Input: part model. Units: mm. Frame: model coordinates. A direction names the side the tool comes from. Coordinates: 2 decimals unless noted, no trailing zeros. Write each loop counter-clockwise with the first axis right and the second up, starting at its lowest first coordinate (ties: lowest second). Pieces come first, ordered by that corner, then holes.
1) Pin query (flat end, axial travel): pin 1 Ø6.5 at (x, y) = (59, 17.5) entering from +Z; pin 2 Ø2 at (y, z) = (20, -56.5) entering from -X; pin 3 Ø7 at (x, z) = (-5, -25.5) entering from +Y. Return the tip coordinate at first contact, or that it passes through.
2) Line query: L1, parallel to Z at x = 19, y = 0.5; L2, parallel to Z at x = -30.5, y = 1; L3, parallel to X at y = 36, z = -3. Output: solid intervals per line, ascending.
3) Section query B-B (z = -55). Output: boundary loops of the cut face in (x, y), then the cut area to 3 significant figures.
4) Section query A-A (z = -25.5). Output: boundary loops of the cut face in (x, y).
5) Set-up query: faces 1 (the flat face through (-47, 18, 10)), 2 (the flat face through (30.036, 7.329, -43.679)), 3 (the flat face through (28.017, 4.827, -46.679)). Return all of +Z, -Z, +X, -X, +Y, -Y with unobstructed straight access to the full face (end or side cutting, diameter ignored); none if empty.
6) Section query C-C (x = 6). Output: boundary loops of the cut face in (y, z).
7) Section query D-D (z = 63.5). Output: boundary loops of the cut face in (x, y), then the cut area to 3 significant figures.
8) Draft query along X for faces 4 (the flat face through (39.46, 11.01, 38.78)), 5 (the flat face through (-40, 12, -80.5)), 6 (the cylindrical face through (55.83, 11.62, -46.69)). Return one class per face: pulls with the +X half, pulls with the -X half, needs draft (parallel to the pull), parting line crosses it, or undercut.
from build123d import *

# Parameters (mm, degrees)
BOSS_EXTRUDE1_DEPTH            = 23
BODY_MOVE_COPY1_ANGLE          = 30
BOSS_EXTRUDE2_DEPTH            = 77.5
BOSS_EXTRUDE2_DEPTH_BACK       = 8.89744
SKETCH13_W                     = 11.5
SKETCH13_H                     = 9.918584287
BOSS_EXTRUDE4_DEPTH            = 31.21169
SHELL1_START                   = 11.5
SHELL1_DEPTH                   = 3
SHELL1_2_DEPTH                 = 22.653212483
SHELL1_3_DEPTH                 = 11.5
SHELL1_4_DEPTH                 = 22.653212483
SHELL1_5_DEPTH                 = 11.5
SHELL1_6_DEPTH                 = 11.153212483
SHELL1_START_2                 = -77.5
SHELL1_7_DEPTH                 = 87.5
SHELL1_START_3                 = -8.897442479
SHELL1_8_DEPTH                 = 86.397442477
SHELL1_START_4                 = -10
SHELL1_9_DEPTH                 = 20
SHELL1_START_5                 = -80.5
SHELL1_10_DEPTH                = 70.5
SHELL1_START_6                 = 10
SHELL1_11_DEPTH                = 70.499999998
SHELL1_START_7                 = -11.897442479
SHELL1_12_DEPTH                = 24.897442479
SHELL1_13_DEPTH                = 3
SHELL1_14_DEPTH                = 3
SHELL1_START_8                 = 77.499999998
SHELL1_15_DEPTH                = 3
SHELL1_16_DEPTH                = 1.897442479
SHELL1_START_9                 = -13
SHELL1_17_DEPTH                = 1.102557521
SHELL1_START_10                = -10.287226583
SHELL1_18_DEPTH                = 1.389784104
CUT_EXTRUDE2_REACH             = 111.579
SKETCH6_R                      = 9
BOSS_EXTRUDE3_DEPTH            = 3
M2_START                       = 36
M2_CLEARANCE_HOLE1_OUTLINE_R   = 1.2
M2_CLEARANCE_HOLE1_DEPTH       = 30.676914536
M2_START_2                     = 63.676914536
M2_CLEARANCE_HOLE1_2_OUTLINE_R = 1.2
M2_CLEARANCE_HOLE1_2_DEPTH     = 3


with BuildPart() as part:
    # Sketch2 → Boss-Extrude1 (new body)
    with BuildSketch(Plane(origin=(0, 0, 0), x_dir=(1, 0, 0), z_dir=(0, 1, 0))):
        Polygon((11, -77.499999998), (34, -77.499999998), (34, -10), (61, -10), (61, 10), (50, 10), (50, 77.5), (27, 77.5), (27, 8.897442479), (11, 8.897442479), align=None)
    extrude(amount=BOSS_EXTRUDE1_DEPTH)


with BuildPart() as part_1:
    # Body-Move/Copy1: moved
    add(part.part.rotate(Axis((36, 15, 0), (0, 0, 1)), BODY_MOVE_COPY1_ANGLE))

    # Sketch7 → Boss-Extrude2 (add, two sides: drawn at the far end of the back side and taken through both)
    with BuildSketch(Plane.XY.offset(-BOSS_EXTRUDE2_DEPTH_BACK)):
        Polygon((10.349364905, 9.42820323), (0, 9.42820323), (0, -10.490381057), (21.849364905, -10.490381057), align=None)
    extrude(amount=BOSS_EXTRUDE2_DEPTH + BOSS_EXTRUDE2_DEPTH_BACK)


with BuildPart() as boss_extrude4_tool:
    # Sketch13 → Boss-Extrude4 (new body)
    with BuildSketch(Plane(origin=(0, 0, -8.897442479), x_dir=(-1, 0, 0), z_dir=(0, 0, -1))):
        with Locations((-5.75, 4.468911087)):
            Rectangle(SKETCH13_W, SKETCH13_H)
    extrude(amount=BOSS_EXTRUDE4_DEPTH)


with BuildPart() as part_2:
    add(part_1.part)


with BuildPart() as part_3:
    # Boss-Extrude4: joined with boss_extrude4_tool
    add(part_2.part.fuse(boss_extrude4_tool.part, tol=0.00001))

    # Shell1: read off the stored shape, not the designer's step
    # Shell1 outline → Shell1 (add)
    with BuildSketch(Plane.YZ.offset(SHELL1_START)):
        Polygon((9.42820323, -13), (9.42820323, -11.897442479), (-3.490381057, -11.897442479), (-3.490381057, -43.109132218), (9.42820323, -43.109132218), align=None)
    extrude(amount=SHELL1_DEPTH)

    # Shell1 2 outline → Shell1 2 (cut)
    with BuildSketch(Plane.YZ):
        Polygon((9.42820323, 13), (9.42820323, 77.499999998), (-10.490381057, 77.499999998), (-10.490381057, -8.897442479), (9.42820323, -8.897442479), (9.42820323, 10), align=None)
    extrude(amount=SHELL1_2_DEPTH, mode=Mode.SUBTRACT)

    # Shell1 3 outline → Shell1 3 (cut)
    with BuildSketch(Plane.YZ):
        Polygon((9.42820323, -10), (9.42820323, -8.897442479), (-0.490381057, -8.897442479), (-0.490381057, -40.109132218), (9.42820323, -40.109132218), (9.42820323, -13), align=None)
    extrude(amount=SHELL1_3_DEPTH, mode=Mode.SUBTRACT)

    # Shell1 4 outline → Shell1 4 (add)
    with BuildSketch(Plane.YZ):
        Polygon((9.42820323, 77.499999998), (9.42820323, 80.499999998), (-13.490381057, 80.499999998), (-13.490381057, -11.897442479), (-0.490381057, -11.897442479), (-0.490381057, -8.897442479), (-10.490381057, -8.897442479), (-10.490381057, 77.499999998), align=None)
    extrude(amount=SHELL1_4_DEPTH)

    # Shell1 5 outline → Shell1 5 (add)
    with BuildSketch(Plane.YZ):
        Polygon((-0.490381057, -11.897442479), (-3.490381057, -11.897442479), (-3.490381057, -43.109132218), (9.42820323, -43.109132218), (9.42820323, -40.109132218), (-0.490381057, -40.109132218), align=None)
    extrude(amount=SHELL1_5_DEPTH)

    # Shell1 6 outline → Shell1 6 (add)
    with BuildSketch(Plane.YZ.offset(SHELL1_START)):
        Polygon((9.42820323, -10), (9.42820323, -8.897442479), (-0.490381057, -8.897442479), (-0.490381057, -11.897442479), (9.42820323, -11.897442479), align=None)
    extrude(amount=SHELL1_6_DEPTH)

    # Shell1 7 outline → Shell1 7 (cut)
    with BuildSketch(Plane.XY.offset(SHELL1_START_2)):
        Polygon((44.124355653, 28.92820323), (24.205771366, 17.42820323), (35.705771366, -2.490381057), (55.624355653, 9.009618943), align=None)
    extrude(amount=SHELL1_7_DEPTH, mode=Mode.SUBTRACT)

    # Shell1 8 outline → Shell1 8 (cut)
    with BuildSketch(Plane.XY.offset(SHELL1_START_3)):
        Polygon((41.767949192, 1.009618943), (30.267949192, 20.92820323), (10.349364905, 9.42820323), (22.653212483, 9.42820323), (22.653212483, -10.026279441), align=None)
    extrude(amount=SHELL1_8_DEPTH, mode=Mode.SUBTRACT)

    # Shell1 9 outline → Shell1 9 (cut)
    with BuildSketch(Plane.XY.offset(SHELL1_START_4)):
        Polygon((44.124355653, 28.92820323), (55.624355653, 9.009618943), (65.150635095, 14.509618943), (53.650635095, 34.42820323), align=None)
    extrude(amount=SHELL1_9_DEPTH, mode=Mode.SUBTRACT)

    # Shell1 11 outline → Shell1 11 (add)
    with BuildSketch(Plane.XY.offset(SHELL1_START_6)):
        Polygon((32.866025404, 22.42820323), (30.267949192, 20.92820323), (41.767949192, 1.009618943), (21.849364905, -10.490381057), (22.653212483, -10.490381057), (22.653212483, -13.490381057), (45.866025404, -0.088457268), align=None)
    extrude(amount=SHELL1_11_DEPTH)



with BuildPart() as body_2:
    # Shell1 10 outline → Shell1 10 (new body)
    with BuildSketch(Plane.XY.offset(SHELL1_START_5)):
        Polygon((55.624355653, 9.009618943), (35.705771366, -2.490381057), (24.205771366, 17.42820323), (21.607695155, 15.92820323), (34.607695155, -6.588457268), (59.722431864, 7.911542732), (46.722431864, 30.42820323), (44.124355653, 28.92820323), align=None)
    extrude(amount=SHELL1_10_DEPTH)


with BuildPart() as part_4:
    add(part_3.part)

    add(body_2.part)  # Shell1 12 merges body 2
    # Shell1 12 outline → Shell1 12 (add)
    with BuildSketch(Plane.XY.offset(SHELL1_START_7)):
        Polygon((21.849364905, -10.490381057), (22.653212483, -10.490381057), (22.653212483, -13.490381057), (69.248711306, 13.411542732), (56.248711306, 35.92820323), (53.650635095, 34.42820323), (65.150635095, 14.509618943), align=None)
    extrude(amount=SHELL1_12_DEPTH)

    # Shell1 13 outline → Shell1 13 (add)
    with BuildSketch(Plane.XY.offset(SHELL1_START_6)):
        Polygon((32.866025404, 22.42820323), (44.366025404, 2.509618943), (65.150635095, 14.509618943), (53.650635095, 34.42820323), align=None)
    extrude(amount=SHELL1_13_DEPTH)

    # Shell1 14 outline → Shell1 14 (add)
    with BuildSketch(Plane.XY.offset(SHELL1_START_5)):
        Polygon((44.124355653, 28.92820323), (24.205771366, 17.42820323), (35.705771366, -2.490381057), (55.624355653, 9.009618943), align=None)
    extrude(amount=SHELL1_14_DEPTH)

    # Shell1 15 outline → Shell1 15 (add)
    with BuildSketch(Plane.XY.offset(SHELL1_START_8)):
        Polygon((41.767949192, 1.009618943), (30.267949192, 20.92820323), (10.349364905, 9.42820323), (22.653212483, 9.42820323), (22.653212483, -10.026279441), align=None)
    extrude(amount=SHELL1_15_DEPTH)

    # Shell1 16 outline → Shell1 16 (add)
    with BuildSketch(Plane.XY.offset(SHELL1_START_7)):
        Polygon((53.650635095, 34.42820323), (46.722431864, 30.42820323), (58.222431864, 10.509618943), (65.150635095, 14.509618943), align=None)
        Polygon((33.107695155, -3.990381057), (21.607695155, 15.92820323), (10.349364905, 9.42820323), (22.653212483, 9.42820323), (22.653212483, -10.026279441), align=None)
    extrude(amount=SHELL1_16_DEPTH)

    # Shell1 17 outline → Shell1 17 (add)
    with BuildSketch(Plane.XY.offset(SHELL1_START_9)):
        Polygon((46.722431864, 30.42820323), (59.722431864, 7.911542732), (69.248711306, 13.411542732), (56.248711306, 35.92820323), align=None)
    extrude(amount=SHELL1_17_DEPTH)

    # Shell1 18 outline → Shell1 18 (add)
    with BuildSketch(Plane.XY.offset(SHELL1_START_10)):
        Polygon((35.705771366, -2.490381057), (24.205771366, 17.42820323), (10.349364905, 9.42820323), (22.653212483, 9.42820323), (22.653212483, -10.026279441), align=None)
    extrude(amount=SHELL1_18_DEPTH)

    # Sketch6 → Cut-Extrude2 (cut, up to next)
    with BuildSketch(Plane(origin=(57.743901834, 33.338457268, 0), x_dir=(0, 0, -1), z_dir=(0.8660254037842566, 0.5000000000003155, 0)), mode=Mode.PRIVATE) as cut_extrude2_sk1:
        with Locations(Location((-67.999999998, -10.009618943, 0), (0, 0, 270))):
            Circle(SKETCH6_R)
    cut_extrude2_tool1 = extrude(cut_extrude2_sk1.sketch, amount=-CUT_EXTRUDE2_REACH, mode=Mode.PRIVATE) & part_4.part
    # Sketch6 → Cut-Extrude2 (cut, up to next)
    with BuildSketch(Plane(origin=(57.743901834, 33.338457268, 0), x_dir=(0, 0, -1), z_dir=(0.8660254037842566, 0.5000000000003155, 0)), mode=Mode.PRIVATE) as cut_extrude2_sk2:
        with Locations(Location((0, -10.509618943, 0), (0, 0, 90))):
            Circle(SKETCH6_R)
    cut_extrude2_tool2 = extrude(cut_extrude2_sk2.sketch, amount=-CUT_EXTRUDE2_REACH, mode=Mode.PRIVATE) & part_4.part
    # Sketch6 → Cut-Extrude2 (cut, up to next)
    with BuildSketch(Plane(origin=(57.743901834, 33.338457268, 0), x_dir=(0, 0, -1), z_dir=(0.8660254037842566, 0.5000000000003155, 0)), mode=Mode.PRIVATE) as cut_extrude2_sk3:
        with Locations(Location((68, -10.009618943, 0), (0, 0, 270))):
            Circle(SKETCH6_R)
    cut_extrude2_tool3 = extrude(cut_extrude2_sk3.sketch, amount=-CUT_EXTRUDE2_REACH, mode=Mode.PRIVATE) & part_4.part
    add(cut_extrude2_tool1.solids().sort_by_distance((62.748711, 24.669873, 68))[0], mode=Mode.SUBTRACT)
    add(cut_extrude2_tool2.solids().sort_by_distance((62.998711, 24.23686, 0))[0], mode=Mode.SUBTRACT)
    add(cut_extrude2_tool3.solids().sort_by_distance((62.748711, 24.669873, -68))[0], mode=Mode.SUBTRACT)

    # Sketch11 → Boss-Extrude3 (add)
    with BuildSketch(Plane(origin=(57.743901834, 33.338457268, 0), x_dir=(0, 0, -1), z_dir=(0.8660254037842566, 0.5000000000003155, 0))):
        Polygon((-13, 2.990381057), (-10, 13.990381057), (10, 13.990381057), (13, 2.990381057), align=None)
    extrude(amount=-BOSS_EXTRUDE3_DEPTH)

    # M2 Clearance Hole1: read off the stored shape, not the designer's step
    # M2 Clearance Hole1 outline → M2 Clearance Hole1 (cut)
    with BuildSketch(Plane(origin=(0, 0, 0), x_dir=(0.5000000000003147, -0.8660254037842569, 0), z_dir=(0.8660254037842569, 0.500000000000315, 0)).offset(M2_START)):
        with Locations((-11.990381057, 8)):
            Circle(M2_CLEARANCE_HOLE1_OUTLINE_R)
        with Locations((-11.990381057, -8)):
            Circle(M2_CLEARANCE_HOLE1_OUTLINE_R)
        with Locations((18.009618943, -75.499999998)):
            Circle(M2_CLEARANCE_HOLE1_OUTLINE_R)
        with Locations((2.009618943, -75.499999998)):
            Circle(M2_CLEARANCE_HOLE1_OUTLINE_R)
        with Locations((18.009618943, -45.499999998)):
            Circle(M2_CLEARANCE_HOLE1_OUTLINE_R)
        with Locations((2.009618943, -45.499999998)):
            Circle(M2_CLEARANCE_HOLE1_OUTLINE_R)
        with Locations((18.009618943, 75.5)):
            Circle(M2_CLEARANCE_HOLE1_OUTLINE_R)
        with Locations((2.009618943, 75.5)):
            Circle(M2_CLEARANCE_HOLE1_OUTLINE_R)
        with Locations((2.009618943, 45.5)):
            Circle(M2_CLEARANCE_HOLE1_OUTLINE_R)
        with Locations((18.009618943, 45.5)):
            Circle(M2_CLEARANCE_HOLE1_OUTLINE_R)
    extrude(amount=M2_CLEARANCE_HOLE1_DEPTH, mode=Mode.SUBTRACT)

    # M2 Clearance Hole1 2 outline → M2 Clearance Hole1 2 (cut)
    with BuildSketch(Plane(origin=(0, 0, 0), x_dir=(0.5000000000003147, -0.8660254037842569, 0), z_dir=(0.8660254037842569, 0.500000000000315, 0)).offset(M2_START_2)):
        with Locations((20.009618943, 10)):
            Circle(M2_CLEARANCE_HOLE1_2_OUTLINE_R)
        with Locations((20.009618943, -10)):
            Circle(M2_CLEARANCE_HOLE1_2_OUTLINE_R)
    extrude(amount=M2_CLEARANCE_HOLE1_2_DEPTH, mode=Mode.SUBTRACT)

    # Mirror1: part across plane


with BuildPart() as part_5:
    add(part_4.part)
    add(part_4.part.mirror(Plane(origin=(0, 0, 0), x_dir=(0, 0, 1), z_dir=(1, 0, 0))))


solid = part_5.part
Answer:
1. pin 1: stops at z = 13
1. pin 2: stops at x = -53.32
1. pin 3: stops at y = -0.49
2. L1: z = -11.9 to -8.9, 77.5 to 80.5
2. L2: z = -80.5 to -8.9, 77.5 to 80.5
2. L3: x = -56.21 to -52.74, 52.74 to 56.21
3. outline: (-59.72, 7.91) - (-34.61, -6.59) - (-21.61, 15.93) - (-24.21, 17.43) - (-35.71, -2.49) - (-55.62, 9.01) - (-44.12, 28.93) - (-46.72, 30.43) - close; (21.61, 15.93) - (34.61, -6.59) - (59.72, 7.91) - (46.72, 30.43) - (44.12, 28.93) - (55.62, 9.01) - (35.71, -2.49) - (24.21, 17.43) - close
3. area: 450 mm2
4. outline: (-59.72, 7.91) - (-34.61, -6.59) - (-21.61, 15.93) - (-24.21, 17.43) - (-35.71, -2.49) - (-55.62, 9.01) - (-44.12, 28.93) - (-46.72, 30.43) - close; (-14.5, -3.49) - (14.5, -3.49) - (14.5, 9.43) - (11.5, 9.43) - (11.5, -0.49) - (-11.5, -0.49) - (-11.5, 9.43) - (-14.5, 9.43) - close; (21.61, 15.93) - (34.61, -6.59) - (59.72, 7.91) - (46.72, 30.43) - (44.12, 28.93) - (55.62, 9.01) - (35.71, -2.49) - (24.21, 17.43) - close
5. face 1: none
5. face 2: +Y
5. face 3: -Z, -Y
6. outline: (-13.49, -11.9) - (-3.49, -11.9) - (-3.49, -43.11) - (9.43, -43.11) - (9.43, -40.11) - (-0.49, -40.11) - (-0.49, -8.9) - (-10.49, -8.9) - (-10.49, 77.5) - (9.43, 77.5) - (9.43, 80.5) - (-13.49, 80.5) - close
7. outline: (-45.87, -0.09) - (-22.65, -13.49) - (22.65, -13.49) - (45.87, -0.09) - (43.26, 4.42) - (40.67, 2.92) - (41.77, 1.01) - (21.85, -10.49) - (-21.85, -10.49) - (-41.77, 1.01) - (-40.67, 2.92) - (-43.26, 4.42) - close; (-35.47, 17.92) - (-32.87, 16.42) - (-30.27, 20.93) - (-32.87, 22.43) - close; (30.27, 20.93) - (32.87, 16.42) - (35.47, 17.92) - (32.87, 22.43) - close
7. area: 336 mm2
8. face 4: pulls with the +X half
8. face 5: needs draft
8. face 6: undercut
